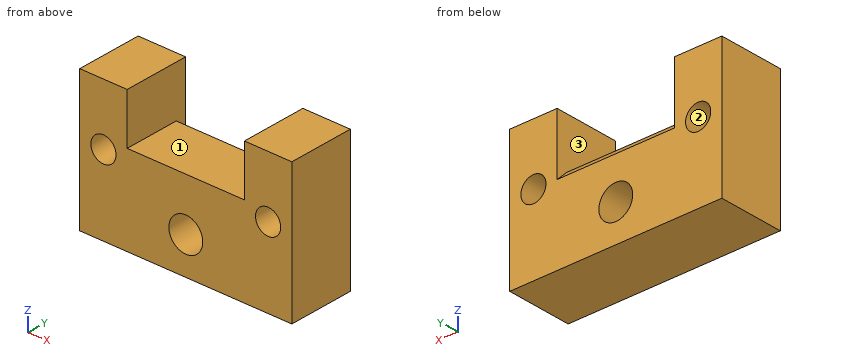
from build123d import *

# Parameters (mm, degrees)
CROQUIS2_W                 = 40.894
CROQUIS2_H                 = 26.924
SALIENTE_EXTRUIR1_DEPTH    = 12.7
CROQUIS3_W                 = 22.606
CROQUIS3_H                 = 9.779
CORTAR_EXTRUIR1_DEPTH      = 12.7
CROQUIS6_R                 = 2.4257
CORTAR_EXTRUIR2_DEPTH      = 12.7
TALADRO_ROSCADO_5_16_181_D = 6.5278
CHAFL_N1_SIZE              = 2.032


with BuildPart() as part:
    # Croquis2 → Saliente-Extruir1 (new body)
    with BuildSketch(Plane(origin=(0, 0, 0), x_dir=(1, 0, 0), z_dir=(0, 1, 0))):
        Rectangle(CROQUIS2_W, CROQUIS2_H)
    extrude(amount=SALIENTE_EXTRUIR1_DEPTH)

    # Croquis3 → Cortar-Extruir1 (cut)
    with BuildSketch(Plane(origin=(0, 12.7, 0), x_dir=(1, 0, 0), z_dir=(0, 1, 0))):
        with Locations((0, -8.5725)):
            Rectangle(CROQUIS3_W, CROQUIS3_H)
    extrude(amount=-CORTAR_EXTRUIR1_DEPTH, mode=Mode.SUBTRACT)

    # Croquis6 → Cortar-Extruir2 (cut)
    with BuildSketch(Plane(origin=(0, 12.7, 0), x_dir=(1, 0, 0), z_dir=(0, 1, 0))):
        with Locations(Location((-15.875, -1.778, 0), (0, 0, 270))):
            Circle(CROQUIS6_R)
        with Locations(Location((15.875, -1.778, 0), (0, 0, 270))):
            Circle(CROQUIS6_R)
    extrude(amount=-CORTAR_EXTRUIR2_DEPTH, mode=Mode.SUBTRACT)

    # Taladro roscado 5/16-181 (through all)
    with Locations(Plane(origin=(0, 12.7, 0), x_dir=(1, 0, 0), z_dir=(0, 1, 0))):
        with Locations((0, 6.35)):
            Hole(TALADRO_ROSCADO_5_16_181_D / 2)

    # Chaflán1
    chafl_n1_edges = [part.edges().sort_by_distance(p)[0] for p in [
        (0, 12.7, 3.683),
    ]]
    chamfer(chafl_n1_edges, length=CHAFL_N1_SIZE)


solid = part.part
Verification items for the finished model (mm, model axes). Face numbers are marked on the shaded views. Coordinates: 2 decimals unless noted, no trailing zeros. Order: outer loops, then holes, each group sorted by start corner. A loop starts at its lowest first (then second) coordinate and runs counter-clockwise, first axis right, second up. Notation, with made-up numbers: M 66.5,-9 L 83.5,-9 A12 ccw 83.5,4 Z; hole C 89.5,33.5 d11. An arc over 180 degrees is marked long. Write each question's results on one line, items separated by ' | '.
1) Section check B-B on z = -6.35. Record the cut outline in (x, y).
Solved:
outline: M -20.45,0 L -3.26,0 L -3.26,12.7 L -20.45,12.7 Z; M 3.26,0 L 20.45,0 L 20.45,12.7 L 3.26,12.7 Z
2) Gauge pin test, flat ends, axial feed: pin 1 Ø5.5 at (x, y) = (-1.5, 4.5) entering from +Z; pin 2 Ø5 at (x, z) = (0, -6.35) entering from -Y. Record the tip position at first contact, or that the pin passes through.
Solved:
pin 1: stops at z = 3.68 | pin 2: passes through
3) Section check C-C on z = 1. Record the cut outline in (x, y), plus the area to 3 significant figures.
Solved:
outline: M -20.45,0 L -18.17,0 L -18.17,12.7 L -20.45,12.7 Z; M -13.58,0 L 13.58,0 L 13.58,12.7 L -13.58,12.7 Z; M 18.17,0 L 20.45,0 L 20.45,12.7 L 18.17,12.7 Z | area: 403 mm²
4) Release check for a two-part mould opening along Z. For the marked faces 1, 2 and 3 record: pulls with the +Z half, pulls with the -Z half, needs draft (parallel to the pull), parting line crosses it, or undercut.
Solved:
face 1: pulls with the +Z half | face 2: undercut | face 3: needs draft
5) Section check D-D on y = 8.75. Record the cut outline in (x, z) (3 decimals).
Solved:
outline: M -20.447,-13.462 L 20.447,-13.462 L 20.447,13.462 L 11.303,13.462 L 11.303,3.683 L -11.303,3.683 L -11.303,13.462 L -20.447,13.462 Z; hole C -15.875,1.778 d4.851; hole C 0,-6.35 d6.528; hole C 15.875,1.778 d4.851
6) Section check A-A on x = 0. Record the cut outline in (y, z).
Solved:
outline: M 0,-13.46 L 12.7,-13.46 L 12.7,-9.61 L 0,-9.61 Z; M 0,-3.09 L 12.7,-3.09 L 12.7,1.65 L 10.67,3.68 L 0,3.68 Z
7) Scan lines: line 1 along X through (y, z) = (10.5, 1.75); line 2 along Z through (x, y) = (0, 10.25); line 3 along Z through (x, y) = (-16, 8). Record each from-to range of solid material in increasing order. Write a range as [from, to].
Solved:
line 1: x = [-20.45, -18.3], [-13.45, 13.45], [18.3, 20.45] | line 2: z = [-13.46, -9.61], [-3.09, 3.68] | line 3: z = [-13.46, -0.64], [4.2, 13.46]
